Part model, mm, in its own coordinate system. A direction names the side the tool comes from. Round coordinates to 2 decimals unless told otherwise and drop trailing zeros. Order: outer loops, then holes, each group sorted by start corner. A loop starts at its lowest first (then second) coordinate and runs counter-clockwise, first axis right, second up. Notation, with made-up numbers: (82, -10.5) - (120, -10.5) arc R20 cw to (120, 26.5) - close; hole circle Ø8 at (-12, -12). An arc over 180 degrees is marked (long way). Answer as a JSON object with one key per item and string values.
```python
from build123d import *

# Parameters (mm, degrees)
CYLINDER095_R            = 4
CYLINDER095_DEPTH        = 20
CYLINDER001_W            = 6
CYLINDER001_H            = 20
CYLINDER001_ANGLE        = 180
CYLINDER003_R            = 1.8
CYLINDER003_DEPTH        = 50
CYLINDER_W               = 9
CYLINDER_H               = 20
CYLINDER_ANGLE           = 170
CYLINDER_PLACEMENT_ANGLE = 5
BOX_W                    = 9
BOX_H                    = 5
BOX_DEPTH                = 20
FILLET_R                 = 6


with BuildPart() as bolt_head_cylinder:
    # Cylinder095 → Cylinder095 (new body)
    with BuildSketch(Plane(origin=(-12, 3, 10), x_dir=(1, 0, 0), z_dir=(0, 1, 0))):
        Circle(CYLINDER095_R)
    extrude(amount=CYLINDER095_DEPTH)


with BuildPart() as top_petals_hole_fusion:
    # Part__Mirroring004: instance of bolt head cylinder
    add(bolt_head_cylinder.part.mirror(Plane(origin=(0, 0, 0), x_dir=(0, -1, 0), z_dir=(1, 0, 0))))

    # Fusion002: union bolt head cylinder
    add(bolt_head_cylinder.part)


with BuildPart() as hole_cylinder:
    # Cylinder001 → Cylinder001 (revolve)
    with BuildSketch(Plane.XZ):
        with Locations((3, 10)):
            Rectangle(CYLINDER001_W, CYLINDER001_H)
    revolve(axis=Axis((0, 0, 0), (0, 0, 1)), revolution_arc=CYLINDER001_ANGLE)


with BuildPart() as bolt_hole:
    # Cylinder003 → Cylinder003 (new body)
    with BuildSketch(Plane(origin=(-12, 20, 10), x_dir=(1, 0, 0), z_dir=(0, -1, 0))):
        Circle(CYLINDER003_R)
    extrude(amount=CYLINDER003_DEPTH)


with BuildPart() as part_mirroring003:
    # Part__Mirroring003: instance of bolt hole
    add(bolt_hole.part.mirror(Plane(origin=(0, 0, 0), x_dir=(0, -1, 0), z_dir=(1, 0, 0))))


with BuildPart() as hole_fusion:
    # Fusion base: copy of bolt hole
    add(bolt_hole.part)

    # Fusion: union hole cylinder, Part__Mirroring003
    add(hole_cylinder.part)
    add(part_mirroring003.part)


with BuildPart() as external_cylinder:
    # Cylinder → Cylinder (revolve)
    with BuildSketch(Plane.XZ):
        with Locations((4.5, 10)):
            Rectangle(CYLINDER_W, CYLINDER_H)
    revolve(axis=Axis((0, 0, 0), (0, 0, 1)), revolution_arc=CYLINDER_ANGLE)


with BuildPart() as external_cylinder_1:
    # Cylinder placement: moved
    add(external_cylinder.part.rotate(Axis((0, 0, 0), (0, 0, 1)), CYLINDER_PLACEMENT_ANGLE))


with BuildPart() as petal_fillet:
    # Box → Box (new body)
    with BuildSketch(Plane(origin=(-15, 1, 0), x_dir=(1, 0, 0), z_dir=(0, 0, 1))):
        with Locations((4.5, 2.5)):
            Rectangle(BOX_W, BOX_H)
    extrude(amount=BOX_DEPTH)

    # Fillet
    fillet_edges = [petal_fillet.edges().sort_by_distance(p)[0] for p in [
        (-15, 3.5, 20),
        (-15, 3.5, 0),
    ]]
    fillet(fillet_edges, radius=FILLET_R)


with BuildPart() as part_mirroring002:
    # Part__Mirroring002: instance of petal fillet
    add(petal_fillet.part.mirror(Plane(origin=(0, 0, 0), x_dir=(0, -1, 0), z_dir=(1, 0, 0))))


with BuildPart() as top_half_cut:
    # Fusion001 base: copy of petal fillet
    add(petal_fillet.part)

    # Fusion001: union external cylinder, Part__Mirroring002
    add(external_cylinder_1.part)
    add(part_mirroring002.part)

    # Cut: cut hole fusion
    add(hole_fusion.part, mode=Mode.SUBTRACT)

    # Cut001: cut top petals hole fusion
    add(top_petals_hole_fusion.part, mode=Mode.SUBTRACT)


solid = top_half_cut.part
```
Item 1: Probe L1, parallel to Y at x = -9, z = 11.25; L2, parallel to Z at x = -12, y = 4.1; L3, parallel to X at y = 5, z = 5.5. List the from-to ranges inside material, lowest first. Write a range as from..to.
Taken from the geometry:
{"L1": "1..3", "L2": "0.8..6, 14..19.2", "L3": "-14.98..-3.32, 3.32..14.98"}
Item 2: Cut at D-D (y = 3.5). Write the cut outline in (x, z).
Taken from the geometry:
{"outline": "(-15, 6) arc R6 ccw to (-9, 0) - (-4.87, 0) - (-4.87, 20) - (-9, 20) arc R6 ccw to (-15, 14) - (-15, 12.65) arc R4 cw (long way) to (-15, 7.35) - close; (4.87, 0) - (9, 0) arc R6 ccw to (15, 6) - (15, 7.35) arc R4 cw (long way) to (15, 12.65) - (15, 14) arc R6 ccw to (9, 20) - (4.87, 20) - close"}
Item 3: Cut at A-A (z = 10). Write the cut outline in (x, y).
Taken from the geometry:
{"outline": "(-15, 1) - (-13.8, 1) - (-13.8, 3) - (-15, 3) - close; (-10.2, 1) - (-8.94, 1) arc R9 ccw to (-8.97, 0.78) - (-5.98, 0.52) arc R6 cw to (5.98, 0.52) - (8.97, 0.78) arc R9 ccw to (8.94, 1) - (10.2, 1) - (10.2, 3) - (8, 3) - (8, 6) - (6.71, 6) arc R9 ccw to (-6.71, 6) - (-8, 6) - (-8, 3) - (-10.2, 3) - close; (13.8, 1) - (15, 1) - (15, 3) - (13.8, 3) - close"}
Item 4: Drop flat-ended pins along their axis: P1, Ø5, axis at x = 12, z = 10, coming from the +Y side; P2, Ø4, axis at x = 10, z = 8.5, coming from the +Y side; P3, Ø6, axis at x = -9, z = 16.5, coming from the +Y side; P4, Ø8, axis at x = -4, z = 9.5, coming from the +Y side. Give the stop position or say it passes through.
Taken from the geometry:
{"P1": "y = 3", "P2": "y = 6", "P3": "y = 6.71", "P4": "y = 9"}
Item 5: Two-plate mould, pull along X, no slides. Class faces 1 (the cylindrical face through (-13.289, 3.535, 18.196)), 2 (the cylindrical face through (12.39, 2.014, 8.243)), 3 (the cylindrical face through (13.289, 3.535, 1.804)): pulls with the +X half, pulls with the -X half, needs draft (parallel to the pull), parting line crosses it, or undercut.
Taken from the geometry:
{"face 1": "pulls with the -X half", "face 2": "undercut", "face 3": "pulls with the +X half"}
Item 6: Tool access for faces 4 (the cylindrical face through (13.289, 3.535, 18.196)), 5 (the cylindrical face through (8, 4, 10)), 6 (the flat face through (7, 6, 10)): list every direction of +Z, -Z, +X, -X, +Y, -Y with a clear straight run to the whole face (end or side of a thin tool).
Taken from the geometry:
{"face 4": "+Z, +X, +Y, -Y", "face 5": "+Y", "face 6": "+Z, -Z, +X, +Y"}
Item 7: Cut at B-B (x = -12). Write the cut outline in (y, z), plus the area to 3 significant figures.
Taken from the geometry:
{"outline": "(1, 0.8) - (6, 0.8) - (6, 6) - (3, 6) - (3, 8.2) - (1, 8.2) - close; (1, 11.8) - (3, 11.8) - (3, 14) - (6, 14) - (6, 19.2) - (1, 19.2) - close", "area": "60.8 mm2"}
Item 8: Cut at C-C (y = 2). Write the cut outline in (x, z).
Taken from the geometry:
{"outline": "(-15, 6) arc R6 ccw to (-9, 0) - (-5.66, 0) - (-5.66, 20) - (-9, 20) arc R6 ccw to (-15, 14) - close; (5.66, 0) - (9, 0) arc R6 ccw to (15, 6) - (15, 14) arc R6 ccw to (9, 20) - (5.66, 20) - close; hole circle Ø3.6 at (-12, 10); hole circle Ø3.6 at (12, 10)"}
